```python
from build123d import *

# Parameters (mm, degrees)
SKETCH1_R           = 76
SKETCH1_R_2         = 27.051
SKETCH1_R_3         = 6.25
BOSS_EXTRUDE1_DEPTH = 4
CUT_EXTRUDE2_DEPTH  = 108.554637278
FILLET1_R           = 5


with BuildPart() as part:
    # Sketch1 → Boss-Extrude1 (new body)
    with BuildSketch(Plane(origin=(0, 0, 0), x_dir=(1, 0, 0), z_dir=(0, 1, 0))):
        with Locations(Location((0, 0, 0), (0, 0, 270))):
            Circle(SKETCH1_R)
        with Locations(Location((0, 0, 0), (0, 0, 270))):
            Circle(SKETCH1_R_2, mode=Mode.SUBTRACT)
        with Locations(Location((0, 62.5, 0), (0, 0, 270))):
            Circle(SKETCH1_R_3, mode=Mode.SUBTRACT)
        with Locations(Location((62.5, 0, 0), (0, 0, 270))):
            Circle(SKETCH1_R_3, mode=Mode.SUBTRACT)
        with Locations(Location((0, -62.5, 0), (0, 0, 270))):
            Circle(SKETCH1_R_3, mode=Mode.SUBTRACT)
        with Locations(Location((-62.5, 0, 0), (0, 0, 270))):
            Circle(SKETCH1_R_3, mode=Mode.SUBTRACT)
    extrude(amount=BOSS_EXTRUDE1_DEPTH)

    # Sketch4 → Cut-Extrude2 (cut, through all)
    with BuildSketch(Plane(origin=(0, 4, 0), x_dir=(1, 0, 0), z_dir=(0, 1, 0))):
        with BuildLine():
            ThreePointArc((-34.504008477, 13.5), (-26.19901335, 26.19901335), (-13.5, 34.504008477))
            Line((-13.5, 34.504008477), (-13.5, 62.5))
            ThreePointArc((-13.5, 62.5), (-45.213382975, 45.213382975), (-62.5, 13.5))
            Line((-62.5, 13.5), (-34.504008477, 13.5))
        make_face()
        with BuildLine():
            ThreePointArc((62.5, 13.5), (45.213382975, 45.213382975), (13.5, 62.5))
            Line((13.5, 62.5), (13.5, 34.504008477))
            ThreePointArc((13.5, 34.504008477), (26.19901335, 26.19901335), (34.504008477, 13.5))
            Line((34.504008477, 13.5), (62.5, 13.5))
        make_face()
        with BuildLine():
            Line((62.5, -13.5), (34.504008477, -13.5))
            ThreePointArc((34.504008477, -13.5), (26.19901335, -26.19901335), (13.5, -34.504008477))
            Line((13.5, -34.504008477), (13.5, -62.5))
            ThreePointArc((13.5, -62.5), (45.213382975, -45.213382975), (62.5, -13.5))
        make_face()
        with BuildLine():
            ThreePointArc((-13.5, -34.504008477), (-26.19901335, -26.19901335), (-34.504008477, -13.5))
            Line((-34.504008477, -13.5), (-62.5, -13.5))
            ThreePointArc((-62.5, -13.5), (-45.213382975, -45.213382975), (-13.5, -62.5))
            Line((-13.5, -62.5), (-13.5, -34.504008477))
        make_face()
    extrude(amount=-CUT_EXTRUDE2_DEPTH, mode=Mode.SUBTRACT)

    # Fillet1
    fillet1_edges = [part.edges().sort_by_distance(p)[0] for p in [
        (-34.504008477, 2, 13.5),
        (-13.5, 2, 34.504008477),
        (-13.5, 2, 62.5),
        (-62.5, 2, 13.5),
        (13.5, 2, 34.504008477),
        (34.504008477, 2, 13.5),
        (62.5, 2, 13.5),
        (13.5, 2, 62.5),
        (34.504008477, 2, -13.5),
        (13.5, 2, -34.504008477),
        (13.5, 2, -62.5),
        (62.5, 2, -13.5),
        (-13.5, 2, -34.504008477),
        (-34.504008477, 2, -13.5),
        (-62.5, 2, -13.5),
        (-13.5, 2, -62.5),
    ]]
    fillet(fillet1_edges, radius=FILLET1_R)


solid = part.part
```
The listing builds one solid part. Answer for the finished solid, in the listing's coordinates (mm). Round coordinates to 2 decimals unless told otherwise and drop trailing zeros. Write each loop counter-clockwise with the first axis right and the second up, starting at its lowest first coordinate (ties: lowest second). Pieces come first, ordered by that corner, then holes. Notation, with made-up numbers: (-1, 49.5) -> (19, 49.5) arc R18 ccw to (19, 58.5) -> close; hole circle Ø4 at (37, -22.5). An arc over 180 degrees is marked (long way). Use CSV: the item, a comma, the result in double quotes. Start each with the question number.
(1) Section B-B on z = 64 is taken. Give the vertices of the cut face in (x, y).
(2) Section A-A on x = 50 is taken. Give the vertices of the cut face in (y, z), then the cut area to 3 significant figures.
(3) Each of these flat-tipped pins is pushed along its axis until it touches: pin 1 (7.5 mm diameter, centred on x = 62.5, z = 0, fed in from +Y); pin 2 (2 mm diameter, centred on x = -42.5, y = 2.5, fed in from -Z); pin 3 (2 mm diameter, centred on x = -44.5, y = 1.5, fed in from +Z); pin 4 (1.5 mm diameter, centred on y = 3.5, z = -60.5, fed in from -X). Where does it stop, or does it pass through?
(4) Section C-C on x = 8 is taken. Give the vertices of the cut face in (y, z).
(5) The mould has two halves that part along X. Classify faces 1 (the face through (-46.245, 1.972, -60.311)), 2 (the face through (1.88, 1.97, -56.54)): released by +X, released by -X, zero draft, split by the parting line, or undercut.
(6) Section D-D on y = 0.8 is taken. Count the separate pieces of the cut face and the enclosed holes in it, then the cut area to 3 significant figures.
(7) Consider L1, parallel to X at y = 1.5, z = 0; L2, parallel to Z at x = 54, y = 0.5; L3, parallel to X at y = 1.3, z = -28. Determine where each line is inside the solid, lowest interval first. Write a range as from..to.
A:
1,outline,"(-40.99, 0) -> (-6.07, 0) -> (-6.07, 4) -> (-40.99, 4) -> close; (6.07, 0) -> (40.99, 0) -> (40.99, 4) -> (6.07, 4) -> close"
2,outline,"(0, -57.24) -> (4, -57.24) -> (4, -39.86) -> (0, -39.86) -> close; (0, -13.5) -> (4, -13.5) -> (4, 13.5) -> (0, 13.5) -> close; (0, 39.86) -> (4, 39.86) -> (4, 57.24) -> (0, 57.24) -> close"
2,area,"247 mm²"
3,pin 1,"passes through"
3,pin 2,"stops at z = -63.67"
3,pin 3,"stops at z = 62.32"
3,pin 4,"stops at x = -46.97"
4,outline,"(0, -75.58) -> (4, -75.58) -> (4, -25.84) -> (0, -25.84) -> close; (0, 25.84) -> (4, 25.84) -> (4, 75.58) -> (0, 75.58) -> close"
5,face 1,"split by the parting line"
5,face 2,"undercut"
6,separate pieces,"1"
6,enclosed holes,"9"
6,area,"9,860 mm²"
7,L1,"x = -76..-68.75, -56.25..-27.05, 27.05..56.25, 68.75..76"
7,L2,"z = -53.48..-34.24, -13.5..13.5, 34.24..53.48"
7,L3,"x = -70.65..-57.48, -24.26..24.26, 57.48..70.65"
